Part model, mm, in its own coordinate system. A direction names the side the tool comes from. Give positions to 0.01 mm unless a question says otherwise; leave off trailing zeros. Order: outer loops, then holes, each group sorted by start corner. A loop starts at its lowest first (then second) coordinate and runs counter-clockwise, first axis right, second up. Notation, with made-up numbers: M 30.5,59.25 L 52.5,59.25 A30 ccw 52.5,87.25 Z; hole C 9,-31 d9. An arc over 180 degrees is marked long. Write each question's results on one line, items separated by ' | '. Start each with the question number.
from build123d import *

# Parameters (mm, degrees)
SKETCH1_R                   = 35
BOSS_EXTRUDE1_DEPTH         = 1.5
BOSS_EXTRUDE2_DEPTH         = 4.6
SKETCH4_R                   = 0.95
CUT_EXTRUDE2_DEPTH          = 7.1
CIRPATTERN5_COUNT           = 2
CIRPATTERN5_ANGLE           = 15
CIRPATTERN6_COUNT           = 2
CIRPATTERN6_ANGLE           = 15
CIRPATTERN1_COUNT           = 5
CIRPATTERN1_COPY_1_SKETCH_R = 0.95
CIRPATTERN1_COPY_1_DEPTH    = 7.1
CIRPATTERN1_COPY_2_SKETCH_R = 0.95
CIRPATTERN1_COPY_2_DEPTH    = 7.1
CIRPATTERN1_COPY_3_SKETCH_R = 0.95
CIRPATTERN1_COPY_3_DEPTH    = 7.1
CIRPATTERN1_COPY_4_SKETCH_R = 0.95
CIRPATTERN1_COPY_4_DEPTH    = 7.1
CIRPATTERN1_COPY_5_SKETCH_R = 0.95
CIRPATTERN1_COPY_5_DEPTH    = 7.1
CIRPATTERN1_COPY_6_SKETCH_R = 0.95
CIRPATTERN1_COPY_6_DEPTH    = 7.1
CIRPATTERN1_COPY_7_SKETCH_R = 0.95
CIRPATTERN1_COPY_7_DEPTH    = 7.1
CIRPATTERN1_COPY_8_SKETCH_R = 0.95
CIRPATTERN1_COPY_8_DEPTH    = 7.1
SKETCH3_R                   = 15
CUT_EXTRUDE1_DEPTH          = 7.1


with BuildPart() as part:
    # Sketch1 → Boss-Extrude1 (new body)
    with BuildSketch(Plane.XY):
        Circle(SKETCH1_R)
    extrude(amount=BOSS_EXTRUDE1_DEPTH)

    # Sketch2 → Boss-Extrude2 (add)
    with BuildSketch(Plane(origin=(0, 0, 0), x_dir=(-1, 0, 0), z_dir=(0, 0, -1))):
        with BuildLine():
            ThreePointArc((-15.56390888, 31.34907878), (0, 21.85), (15.56390888, 31.34907878))
            ThreePointArc((15.56390888, 31.34907878), (0, 35), (-15.56390888, 31.34907878))
        make_face()
    boss_extrude2 = extrude(amount=BOSS_EXTRUDE2_DEPTH)

    # Sketch4 → Cut-Extrude2 (cut, through all)
    with BuildSketch(Plane.XY.offset(1.5)):
        with Locations((0, 32)):
            Circle(SKETCH4_R)
    cut_extrude2 = extrude(amount=-CUT_EXTRUDE2_DEPTH, mode=Mode.SUBTRACT)

    # CirPattern5: Cut-Extrude2 ×2 about axis
    cirpattern5_axis = Axis((0, 0, -88.99), (0, 0, 1))
    for i in range(1, CIRPATTERN5_COUNT):
        add(cut_extrude2.rotate(cirpattern5_axis, i * CIRPATTERN5_ANGLE / (CIRPATTERN5_COUNT - 1)), mode=Mode.SUBTRACT)

    # CirPattern6: Cut-Extrude2 ×2 about axis
    cirpattern6_axis = Axis((0, 0, -88.99), (0, 0, -1))
    for i in range(1, CIRPATTERN6_COUNT):
        add(cut_extrude2.rotate(cirpattern6_axis, i * CIRPATTERN6_ANGLE / (CIRPATTERN6_COUNT - 1)), mode=Mode.SUBTRACT)

    # CirPattern1: Boss-Extrude2, Cut-Extrude2 ×5 about axis
    cirpattern1_axis = Axis((0, 0, 0), (0, 0, 1))
    for i in range(1, CIRPATTERN1_COUNT):
        add(boss_extrude2.rotate(cirpattern1_axis, i * 360 / CIRPATTERN1_COUNT))
        add(cut_extrude2.rotate(cirpattern1_axis, i * 360 / CIRPATTERN1_COUNT), mode=Mode.SUBTRACT)

    # CirPattern1 copy 1 sketch → CirPattern1 copy 1 (cut, through all)
    with BuildSketch(Plane(origin=(0, 0, 1.5), x_dir=(0.052335956, 0.998629535, 0), z_dir=(0, 0, 1))):
        with Locations((0, 32)):
            Circle(CIRPATTERN1_COPY_1_SKETCH_R)
    extrude(amount=-CIRPATTERN1_COPY_1_DEPTH, mode=Mode.SUBTRACT)

    # CirPattern1 copy 2 sketch → CirPattern1 copy 2 (cut, through all)
    with BuildSketch(Plane(origin=(0, 0, 1.5), x_dir=(-0.933580426, 0.35836795, 0), z_dir=(0, 0, 1))):
        with Locations((0, 32)):
            Circle(CIRPATTERN1_COPY_2_SKETCH_R)
    extrude(amount=-CIRPATTERN1_COPY_2_DEPTH, mode=Mode.SUBTRACT)

    # CirPattern1 copy 3 sketch → CirPattern1 copy 3 (cut, through all)
    with BuildSketch(Plane(origin=(0, 0, 1.5), x_dir=(-0.629320391, -0.777145961, 0), z_dir=(0, 0, 1))):
        with Locations((0, 32)):
            Circle(CIRPATTERN1_COPY_3_SKETCH_R)
    extrude(amount=-CIRPATTERN1_COPY_3_DEPTH, mode=Mode.SUBTRACT)

    # CirPattern1 copy 4 sketch → CirPattern1 copy 4 (cut, through all)
    with BuildSketch(Plane(origin=(0, 0, 1.5), x_dir=(0.544639035, -0.838670568, 0), z_dir=(0, 0, 1))):
        with Locations((0, 32)):
            Circle(CIRPATTERN1_COPY_4_SKETCH_R)
    extrude(amount=-CIRPATTERN1_COPY_4_DEPTH, mode=Mode.SUBTRACT)

    # CirPattern1 copy 5 sketch → CirPattern1 copy 5 (cut, through all)
    with BuildSketch(Plane(origin=(0, 0, 1.5), x_dir=(0.544639035, 0.838670568, 0), z_dir=(0, 0, 1))):
        with Locations((0, 32)):
            Circle(CIRPATTERN1_COPY_5_SKETCH_R)
    extrude(amount=-CIRPATTERN1_COPY_5_DEPTH, mode=Mode.SUBTRACT)

    # CirPattern1 copy 6 sketch → CirPattern1 copy 6 (cut, through all)
    with BuildSketch(Plane(origin=(0, 0, 1.5), x_dir=(-0.629320391, 0.777145961, 0), z_dir=(0, 0, 1))):
        with Locations((0, 32)):
            Circle(CIRPATTERN1_COPY_6_SKETCH_R)
    extrude(amount=-CIRPATTERN1_COPY_6_DEPTH, mode=Mode.SUBTRACT)

    # CirPattern1 copy 7 sketch → CirPattern1 copy 7 (cut, through all)
    with BuildSketch(Plane(origin=(0, 0, 1.5), x_dir=(-0.933580426, -0.35836795, 0), z_dir=(0, 0, 1))):
        with Locations((0, 32)):
            Circle(CIRPATTERN1_COPY_7_SKETCH_R)
    extrude(amount=-CIRPATTERN1_COPY_7_DEPTH, mode=Mode.SUBTRACT)

    # CirPattern1 copy 8 sketch → CirPattern1 copy 8 (cut, through all)
    with BuildSketch(Plane(origin=(0, 0, 1.5), x_dir=(0.052335956, -0.998629535, 0), z_dir=(0, 0, 1))):
        with Locations((0, 32)):
            Circle(CIRPATTERN1_COPY_8_SKETCH_R)
    extrude(amount=-CIRPATTERN1_COPY_8_DEPTH, mode=Mode.SUBTRACT)

    # Sketch3 → Cut-Extrude1 (cut, through all)
    with BuildSketch(Plane.XY.offset(1.5)):
        Circle(SKETCH3_R)
    extrude(amount=-CUT_EXTRUDE1_DEPTH, mode=Mode.SUBTRACT)


solid = part.part
(1) Pull direction X, two halves, no side cores. Call faces 1 (the cylindrical face through (-10.557, -29.605, -1.507)), 2 (the flat face through (7, -15, 1.5)): +X half, -X half, draft (parallel to the pull), parting line (faces both ways), or undercut.
(2) Probe L1, parallel to X at y = -20.5, z = -3.25; L2, parallel to X at y = -26, z = -3.75; L3, parallel to Y at x = 24.5, z = -0.5 (3 decimals). List the from-to ranges inside material, lowest first.
(3) Saw through at A-A on x = 0. Give the cut face in (y, z).
(4) Drop flat-ended pins along their axis: P1, Ø2, axis at x = -18.5, z = -2.5, coming from the +Y side; P2, Ø3, axis at x = 8.28, y = 30.91, coming from the +Z side; P3, Ø3, axis at y = -23, z = -3, coming from the +X side; P4, Ø2, axis at x = 22, y = -1, coming from the -Z side. Give the stop position or say it passes through.
(5) Saw through at C-C on y = -3. Give the cut face in (x, z), plus the area to 3 significant figures.
(6) Tool access for faces 3 (the cylindrical face through (0.268, 21.852, -2.268)), 4 (the flat face through (-27, 9, -4.6)): list every direction of +Z, -Z, +X, -X, +Y, -Y with a clear straight run to the whole face (end or side of a thin tool).
(7) Saw through at D-D on y = 23. Give the cut face in (x, z).
(8) Saw through at B-B on z = -1.25. Give the number of separate pieces and of enclosed holes in the cut face, plus the area to 3 significant figures.
Taken from the geometry:
1) face 1: undercut | face 2: draft
2) L1: x = -28.37 to -25.75, -23.99 to -9.8, 9.8 to 23.99, 25.75 to 28.37 | L2: x = -23.43 to -19.75, -17.87 to -6.63, 6.63 to 17.87, 19.75 to 23.43 | L3: y = -24.995 to -21.014, -19.263 to -14.389, 0.361 to 23.959
3) outline: M -35,0 L -15,0 L -15,1.5 L -35,1.5 Z; M 15,0 L 21.85,0 L 21.85,-4.6 L 31.05,-4.6 L 31.05,1.5 L 15,1.5 Z; M 32.95,-4.6 L 35,-4.6 L 35,1.5 L 32.95,1.5 Z
4) P1: stops at y = -14.72 | P2: stops at z = 1.5 | P3: stops at x = 27.62 | P4: stops at z = 0
5) outline: M -34.87,-4.6 L -28.68,-4.6 L -28.68,0 L -14.7,0 L -14.7,1.5 L -34.87,1.5 Z; M 14.7,0 L 28.68,0 L 28.68,-4.6 L 34.87,-4.6 L 34.87,1.5 L 14.7,1.5 Z | area: 117 mm²
6) face 3: -Z | face 4: -Z, +X, -X, +Y, -Y
7) outline: M -26.38,-4.6 L -23.69,-4.6 L -23.69,0 L -6.24,0 L -6.24,-4.6 L 6.24,-4.6 L 6.24,0 L 23.69,0 L 23.69,-4.6 L 26.38,-4.6 L 26.38,1.5 L -26.38,1.5 Z
8) separate pieces: 5 | enclosed holes: 15 | area: 1,400 mm²
